from build123d import *

# Parameters (mm, degrees)
SKETCH1_W           = 320
SKETCH1_H           = 110
SKETCH1_R           = 2.25
BOSS_EXTRUDE1_DEPTH = 5
SKETCH2_W           = 320
SKETCH2_H           = 105
SKETCH2_R           = 2.25
BOSS_EXTRUDE2_DEPTH = 3
CHAMFER1_SIZE       = 8
CHAMFER3_SIZE       = 3
SKETCH3_W           = 7.071067812
SKETCH3_H           = 2.6
CUT_EXTRUDE1_DEPTH  = 357.223151056


with BuildPart() as part:
    # Sketch1 → Boss-Extrude1 (new body)
    with BuildSketch(Plane.XY):
        with Locations((160, 55)):
            Rectangle(SKETCH1_W, SKETCH1_H)
        with Locations((20, 9)):
            Circle(SKETCH1_R, mode=Mode.SUBTRACT)
        with Locations(Location((300, 9, 0), (0, 0, 180))):
            Circle(SKETCH1_R, mode=Mode.SUBTRACT)
        with Locations((20, 98)):
            Circle(SKETCH1_R, mode=Mode.SUBTRACT)
        with Locations(Location((300, 98, 0), (0, 0, 180))):
            Circle(SKETCH1_R, mode=Mode.SUBTRACT)
    extrude(amount=-BOSS_EXTRUDE1_DEPTH)

    # Sketch2 → Boss-Extrude2 (add)
    with BuildSketch(Plane(origin=(0, 0, -5), x_dir=(-1, 0, 0), z_dir=(0, 0, -1))):
        with Locations((-160, 57.5)):
            Rectangle(SKETCH2_W, SKETCH2_H)
        with Locations(Location((-20, 9, 0), (0, 0, 180))):
            Circle(SKETCH2_R, mode=Mode.SUBTRACT)
        with Locations((-300, 9)):
            Circle(SKETCH2_R, mode=Mode.SUBTRACT)
        with Locations(Location((-20, 98, 0), (0, 0, 180))):
            Circle(SKETCH2_R, mode=Mode.SUBTRACT)
        with Locations((-300, 98)):
            Circle(SKETCH2_R, mode=Mode.SUBTRACT)
    extrude(amount=BOSS_EXTRUDE2_DEPTH)

    # Chamfer1
    # the kernel refuses this chamfer: 8 mm, written as the material it takes off along each edge
    with BuildSketch(Plane(origin=(320, -15.573463904, -8), x_dir=(-0.9996219169112968, 0, -0.0274958766105862), z_dir=(0, 1, 0)), Plane(origin=(0, 130.573463904, -8), x_dir=(0.9996219169112968, 0, -0.027495876610586275), z_dir=(0, -1, 0))) as chamfer1_piece_1:
        Polygon((CHAMFER1_SIZE * 0.999621916911, CHAMFER1_SIZE * 0.0274958766106), (-CHAMFER1_SIZE * 0.0274958766106, CHAMFER1_SIZE * 0.999621916911), (0, 0), align=None)
    extrude(amount=146.146927807, mode=Mode.SUBTRACT)

    # Chamfer3
    chamfer3_edges = [part.edges().sort_by_distance(p)[0] for p in [
        (160, 110, -8),
    ]]
    chamfer(chamfer3_edges, length=CHAMFER3_SIZE)

    # Sketch3 → Cut-Extrude1 (cut, through all, along a direction that is not the sketch's normal)
    with BuildSketch(Plane(origin=(160, 0, -160), x_dir=(-0.7071067811865452, 0, -0.7071067811865498), z_dir=(0.7071067811865498, 0, -0.7071067811865452))):
        with Locations((-222.738636074, 1.3)):
            Rectangle(SKETCH3_W, SKETCH3_H)
    extrude(amount=-CUT_EXTRUDE1_DEPTH, dir=(1, 0, 0), mode=Mode.SUBTRACT)


solid = part.part
The listing builds one solid part. Answer for the finished solid, in the listing's coordinates (mm). Give positions to 0.01 mm unless a question says otherwise; leave off trailing zeros. Write each loop counter-clockwise with the first axis right and the second up, starting at its lowest first coordinate (ties: lowest second). Pieces come first, ordered by that corner, then holes.
Item 1: Flat-ended cylindrical pins translate along their axes: P1, Ø1, axis at y = 27, z = -6.5, coming from the +X side; P2, Ø2.5, axis at x = 228.5, y = 3.5, coming from the -Z side; P3, Ø3, axis at y = 20.5, z = -5.5, coming from the -X side. Find the tip coordinate at first contact, or state that the pin passes through.
Item 2: Section A-A, the plane z = -3.5 is taken. Write down the section's boundary in (x, y).
Item 3: Find the intervals of material crossed by line 1 along Y through (x, z) = (20, -1.8); line 2 along Y through (x, z) = (300, -6.15); line 3 along X through (y, z) = (98, -7.2), in increasing order.
Item 4: Section B-B, the plane y = 62 is taken. Write down the section's boundary in (x, z).
Completed:
1. P1: stops at x = 314
1. P2: stops at z = -5
1. P3: stops at x = 4
2. outline: (3.5, 2.6) - (316.5, 2.6) - (316.5, 110) - (3.5, 110) - close; hole circle Ø4.5 at (20, 9); hole circle Ø4.5 at (20, 98); hole circle Ø4.5 at (300, 9); hole circle Ø4.5 at (300, 98)
3. line 1: y = 2.6 to 6.75, 11.25 to 95.75, 100.25 to 110
3. line 2: y = 5 to 6.75, 11.25 to 95.75, 100.25 to 108.85
3. line 3: x = 7.2 to 17.75, 22.25 to 297.75, 302.25 to 312.8
4. outline: (0, 0) - (8, -8) - (312, -8) - (320, 0) - close
